```python
from build123d import *

# Parameters (mm, degrees)
ESQUISSE1_W             = 13
ESQUISSE1_H             = 18
EXTRUSION1_DEPTH        = 10
ESQUISSE2_R             = 5
ENL_V_MAT_EXTRU_1_DEPTH = 11


with BuildPart() as part:
    # Esquisse1 → Extrusion1 (new body)
    with BuildSketch(Plane(origin=(0, 0, 0), x_dir=(0, 0, -1), z_dir=(1, 0, 0))):
        with Locations((6.5, 9)):
            Rectangle(ESQUISSE1_W, ESQUISSE1_H)
    extrude(amount=EXTRUSION1_DEPTH)

    # Esquisse2 → Enlèv. mat.-Extru.1 (cut, through all)
    with BuildSketch(Plane.ZY):
        with Locations((-5.5, 9)):
            Circle(ESQUISSE2_R)
    extrude(amount=-ENL_V_MAT_EXTRU_1_DEPTH, mode=Mode.SUBTRACT)


solid = part.part
```
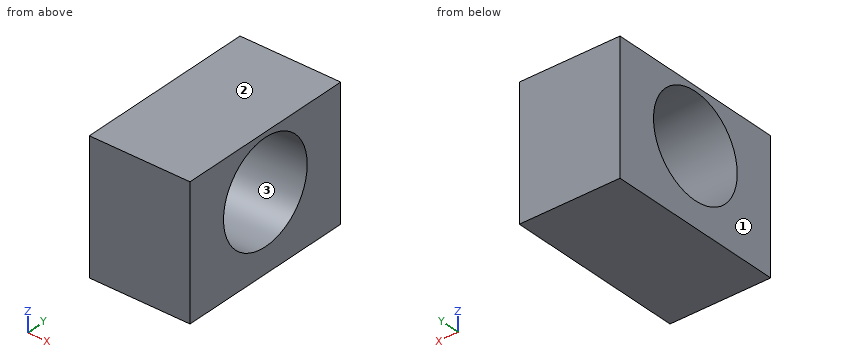
Part model, mm, in its own coordinate system. Face numbers are marked on the shaded views. Round coordinates to 2 decimals unless told otherwise and drop trailing zeros. Loops run counter-clockwise (first coordinate to the right, second up) from the corner with the lowest first, then second, coordinate; pieces in that order, holes last.
1. Two-plate mould, pull along Z, no slides. Class the marked faces 1, 2 and 3: pulls with the +Z half, pulls with the -Z half, needs draft (parallel to the pull), parting line crosses it, or undercut.
Solutions:
face 1: needs draft
face 2: pulls with the +Z half
face 3: undercut
2. Slice it at C-C (x = 3.75). Give the cut face in (y, z).
Solutions:
outline: (0, -13) - (18, -13) - (18, 0) - (0, 0) - close; hole circle Ø10 at (9, -5.5)
3. Slice it at B-B (z = -5.5). Give the cut face in (x, y).
Solutions:
outline: (0, 0) - (10, 0) - (10, 4) - (0, 4) - close; (0, 14) - (10, 14) - (10, 18) - (0, 18) - close
4. Drill centre lines: line 1 along Y through (x, z) = (5.75, -5.5); line 2 along Y through (x, z) = (1, -1); line 3 along Z through (x, y) = (6.5, 8.75). Where is each one in solid material? Low to high.
Solutions:
line 1: y = 0 to 4, 14 to 18
line 2: y = 0 to 6.82, 11.18 to 18
line 3: z = -13 to -10.49, -0.51 to 0
5. Slice it at A-A (y = 9). Give the cut face in (x, z).
Solutions:
outline: (0, -13) - (10, -13) - (10, -10.5) - (0, -10.5) - close; (0, -0.5) - (10, -0.5) - (10, 0) - (0, 0) - close
